from build123d import *

# Parameters (mm, degrees)
SKETCH1_W                      = 152.4
SKETCH1_H                      = 63.5
BOSS_EXTRUDE1_DEPTH            = 3.175
EDGE_FLANGE1_STRIP_W           = 25.4
EDGE_FLANGE1_STRIP_H           = 3.175
EDGE_FLANGE1_STRIP_CUT_DEPTH   = 63.5
EDGE_FLANGE1_STRIP_2_W         = 25.4
EDGE_FLANGE1_STRIP_2_H         = 3.175
EDGE_FLANGE1_STRIP_CUT_2_DEPTH = 63.5
EDGE_FLANGE1_DEPTH             = 63.5
EDGE_FLANGE1_BEND_DEPTH        = 63.5
CUT_EXTRUDE1_DEPTH             = 194.857086535
CUT_EXTRUDE1_DEPTH_BACK        = 194.857086535
SKETCH22_R                     = 3.175


# Sheet-metal steps are written as plain solids
with BuildPart() as part:
    # Sketch1 → Boss-Extrude1 (new body)
    with BuildSketch(Plane.XY):
        with Locations((76.2, 31.75)):
            Rectangle(SKETCH1_W, SKETCH1_H)
    extrude(amount=BOSS_EXTRUDE1_DEPTH)

    # Edge-Flange1 strip (across the edge) → Edge-Flange1 strip cut (cut)
    with BuildSketch(Plane(origin=(0, 63.5, 3.175), x_dir=(1, 0, 0), z_dir=(0, -1, 0))):
        with Locations((-3.175, -1.5875)):
            Rectangle(EDGE_FLANGE1_STRIP_W, EDGE_FLANGE1_STRIP_H)
    extrude(amount=EDGE_FLANGE1_STRIP_CUT_DEPTH, mode=Mode.SUBTRACT)

    # Edge-Flange1 strip 2 (across the edge) → Edge-Flange1 strip cut 2 (cut)
    with BuildSketch(Plane(origin=(152.4, 0, 3.175), x_dir=(-1, 0, 0), z_dir=(0, 1, 0))):
        with Locations((-3.175, -1.5875)):
            Rectangle(EDGE_FLANGE1_STRIP_2_W, EDGE_FLANGE1_STRIP_2_H)
    extrude(amount=EDGE_FLANGE1_STRIP_CUT_2_DEPTH, mode=Mode.SUBTRACT)

    # Edge-Flange1 section (across the edge) → Edge-Flange1 (add)
    with BuildSketch(Plane(origin=(0, 63.5, 3.175), x_dir=(1, 0, 0), z_dir=(0, -1, 0))):
        with BuildLine():
            Line((0, 6.35), (0, 98.425))
            Line((0, 98.425), (3.175, 98.425))
            Line((3.175, 98.425), (3.175, 6.35))
            ThreePointArc((3.175, 6.35), (5.034871939, 1.859871939), (9.525, 0))
            Line((9.525, 0), (9.525, -3.175))
            ThreePointArc((9.525, -3.175), (2.789807909, -0.385192091), (0, 6.35))
        make_face()
    extrude(amount=EDGE_FLANGE1_DEPTH)

    # Edge-Flange1 section 2 (across the edge) → Edge-Flange1 bend (add)
    with BuildSketch(Plane(origin=(152.4, 0, 3.175), x_dir=(-1, 0, 0), z_dir=(0, 1, 0))):
        with BuildLine():
            Line((0, 6.35), (0, 98.425))
            Line((0, 98.425), (3.175, 98.425))
            Line((3.175, 98.425), (3.175, 6.35))
            ThreePointArc((3.175, 6.35), (5.034871939, 1.859871939), (9.525, 0))
            Line((9.525, 0), (9.525, -3.175))
            ThreePointArc((9.525, -3.175), (2.789807909, -0.385192091), (0, 6.35))
        make_face()
    extrude(amount=EDGE_FLANGE1_BEND_DEPTH)

    # Sketch22 → Cut-Extrude1 (cut, two sides: drawn at the far end of the back side and taken through both)
    with BuildSketch(Plane.ZY.offset(-CUT_EXTRUDE1_DEPTH_BACK)):
        with Locations((50.8, 15.24)):
            Circle(SKETCH22_R)
    extrude(amount=CUT_EXTRUDE1_DEPTH + CUT_EXTRUDE1_DEPTH_BACK, mode=Mode.SUBTRACT)


solid = part.part
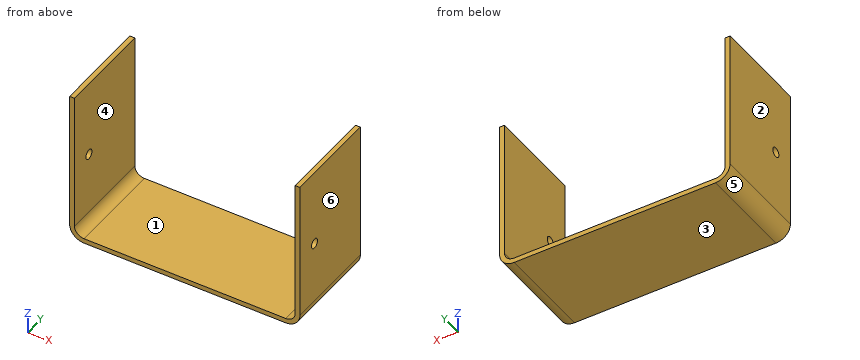
Work out the finished part from the listing and answer in its coordinate system (mm). Face numbers are marked on the shaded views. A direction names the side the tool comes from. Give positions to 0.01 mm unless a question says otherwise; leave off trailing zeros. Loops run counter-clockwise (first coordinate to the right, second up) from the corner with the lowest first, then second, coordinate; pieces in that order, holes last. Notation, with made-up numbers: (56, 66.25) - (113, 66.25) arc R22 ccw to (113, 85.25) - close; hole circle Ø8 at (44.25, -7). An arc over 180 degrees is marked (long way). Answer in a Markdown table with one row per item.
(1) Consider L1, parallel to Y at x = 1.3, z = 50.8 (3 decimals); L2, parallel to X at y = 47.5, z = 52.5 (3 decimals); L3, parallel to Z at x = 150, y = 15. Determine where each line is inside the solid, lowest interval first. Write a range as [from, to].
Results list:
| item | result |
|---|---|
| L1 | y = [0, 12.065], [18.415, 63.5] |
| L2 | x = [0, 3.175], [149.225, 152.4] |
| L3 | z = [3.2, 47.63], [53.97, 101.6] |
(2) For a pull along X with two mould halves and no side action, classify the marked faces 3, 4, 5 and 6 as pulls with the +X half, pulls with the -X half, needs draft (parallel to the pull), parting line crosses it, or undercut.
Results list:
| item | result |
|---|---|
| face 3 | needs draft |
| face 4 | undercut |
| face 5 | pulls with the -X half |
| face 6 | pulls with the +X half |
(3) Section C-C (z = 50.8) is taken. Give the vertices of the cut face in (x, y) (3 decimals), and give its area (3 significant figures).
Results list:
| item | result |
|---|---|
| outline | (0, 0) - (3.175, 0) - (3.175, 12.065) - (0, 12.065) - close; (0, 18.415) - (3.175, 18.415) - (3.175, 63.5) - (0, 63.5) - close; (149.225, 0) - (152.4, 0) - (152.4, 12.065) - (149.225, 12.065) - close; (149.225, 18.415) - (152.4, 18.415) - (152.4, 63.5) - (149.225, 63.5) - close |
| area | 363 mm² |
(4) A tool of negligible diameter and unlimited length cuts with its end or side. For the marked faces 1 and 2, from which of +Z, -Z, +X, -X, +Y, -Y can it reach the whole face along a straight path? Write none if from no direction.
Results list:
| item | result |
|---|---|
| face 1 | +Z, +Y, -Y |
| face 2 | +Z, -Z, -X, +Y, -Y |
(5) Section B-B (z = 35) is taken. Give the vertices of the cut face in (x, y) (3 decimals), and give its area (3 significant figures).
Results list:
| item | result |
|---|---|
| outline | (0, 0) - (3.175, 0) - (3.175, 63.5) - (0, 63.5) - close; (149.225, 0) - (152.4, 0) - (152.4, 63.5) - (149.225, 63.5) - close |
| area | 403 mm² |
(6) Section D-D (y = 4.5) is taken. Give the vertices of the cut face in (x, z) (3 decimals).
Results list:
| item | result |
|---|---|
| outline | (0, 9.525) arc R9.525 ccw to (9.525, 0) - (142.875, 0) arc R9.525 ccw to (152.4, 9.525) - (152.4, 101.6) - (149.225, 101.6) - (149.225, 9.525) arc R6.35 cw to (142.875, 3.175) - (9.525, 3.175) arc R6.35 cw to (3.175, 9.525) - (3.175, 101.6) - (0, 101.6) - close |
(7) Section A-A (y = 15.24) is taken. Give the vertices of the cut face in (x, z) (3 decimals), and give its area (3 significant figures).
Results list:
| item | result |
|---|---|
| outline | (0, 9.525) arc R9.525 ccw to (9.525, 0) - (142.875, 0) arc R9.525 ccw to (152.4, 9.525) - (152.4, 47.625) - (149.225, 47.625) - (149.225, 9.525) arc R6.35 cw to (142.875, 3.175) - (9.525, 3.175) arc R6.35 cw to (3.175, 9.525) - (3.175, 47.625) - (0, 47.625) - close; (0, 53.975) - (3.175, 53.975) - (3.175, 101.6) - (0, 101.6) - close; (149.225, 53.975) - (152.4, 53.975) - (152.4, 101.6) - (149.225, 101.6) - close |
| area | 1,050 mm² |
(8) A flat-ended cylindrical pin translates along its axis: pin 1 Ø1 at (x, y) = (21.5, 23) entering from +Z (3 decimals). Find the tip coordinate at first contact, or state that the pin passes through.
Results list:
| item | result |
|---|---|
| pin 1 | stops at z = 3.175 |
